Here's how the part is built. I have some questions about the finished solid (model axes, mm). Face numbers are marked on the shaded views. A direction names the side the tool comes from. Coordinates: 2 decimals unless noted, no trailing zeros. Loops run counter-clockwise (first coordinate to the right, second up) from the corner with the lowest first, then second, coordinate; pieces in that order, holes last. Notation, with made-up numbers: (69, 17.25) -> (114, 17.25) arc R23 ccw to (114, 48.25) -> close; hole circle Ø10 at (64, 33). An arc over 180 degrees is marked (long way). Use CSV: the item, a comma, the result in double quotes. Start each with the question number.
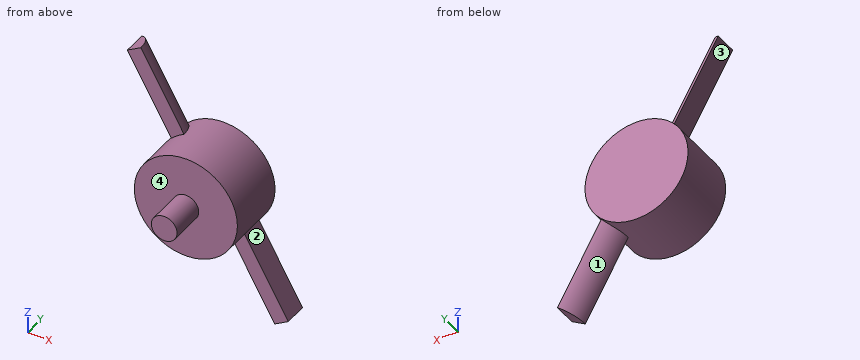
from build123d import *

# Parameters (mm, degrees)
F0_R         = 10
F1_DEPTH     = 12
F3_DEPTH     = 5
F4_T4_DEPTH  = 41.8533803035
F4_S5_R      = 10
F4_T6_DEPTH  = 25
F4_T10_DEPTH = 41.8533803035
F4_S11_R     = 10
F4_T12_DEPTH = 25
F5_R         = 2.5
F6_DEPTH     = 6.9


# Not quite as in the source:
# - a fillet or chamfer that OpenCascade refuses, or shapes differently, is made with other operations: its cross-section is extruded or revolved along the edge and cut away or added


with BuildPart() as f1:
    # F0 (on Front) → F1 (new body)
    with BuildSketch(Plane.XZ):
        Circle(F0_R)
    extrude(amount=F1_DEPTH)

    # F2 (on face) → F3 (join)
    with BuildSketch(Plane(origin=(0, 0, 0), x_dir=(-1, 0, 0), z_dir=(0, 1, 0))):
        Polygon((2.4069448783, 5), (-2.4069448783, 5), (-3, 0), (3, 0), (15.6031129395, 22), (13, 23.4912421078), align=None)
        Polygon((3, 0), (-3, 0), (-15.6031129395, -22), (-13, -23.4912421078), (-2.4069448783, -5), (2.4069448783, -5), align=None)
    extrude(amount=-F3_DEPTH)

    # F4: fillet of radius 5 on 2 edges, made by hand


with BuildPart() as f4_tool2:
    # F4_s3 → F4_t4 (new body)
    with BuildSketch(Plane(origin=(-19.5578893967, 0, 34.1402611236), x_dir=(0, 1, 0), z_dir=(0.4970807026, 0, -0.8677043132))):
        with BuildLine():
            ThreePointArc((0, -4.6031129395), (-1.4644660941, -1.0675790336), (-5, 0.3968870605))
            Line((-5, 0.3968870605), (0, 0.3968870605))
            Line((0, 0.3968870605), (0, -4.6031129395))
        make_face()
    extrude(amount=F4_T4_DEPTH)

    # F4_s5 → F4_t6 (cut, symmetric)
    with BuildSketch(Plane.XZ.offset(2.5)):
        Circle(F4_S5_R)
    extrude(amount=F4_T6_DEPTH, both=True, mode=Mode.SUBTRACT)


with BuildPart() as f1_1:
    add(f1.part)

    # F4_t1: cut F4_tool2
    add(f4_tool2.part, mode=Mode.SUBTRACT)


with BuildPart() as f4_tool8:
    # F4_s9 → F4_t10 (new body)
    with BuildSketch(Plane(origin=(19.5578893967, 0, -34.1402611236), x_dir=(0, 1, 0), z_dir=(-0.4970807026, 0, 0.8677043132))):
        with BuildLine():
            ThreePointArc((0, -4.6031129395), (-1.4644660941, -1.0675790336), (-5, 0.3968870605))
            Line((-5, 0.3968870605), (0, 0.3968870605))
            Line((0, 0.3968870605), (0, -4.6031129395))
        make_face()
    extrude(amount=F4_T10_DEPTH)

    # F4_s11 → F4_t12 (cut, symmetric)
    with BuildSketch(Plane.XZ.offset(2.5)):
        Circle(F4_S11_R)
    extrude(amount=F4_T12_DEPTH, both=True, mode=Mode.SUBTRACT)


with BuildPart() as f1_2:
    add(f1_1.part)

    # F4_t7: cut F4_tool8
    add(f4_tool8.part, mode=Mode.SUBTRACT)

    # F5 (on face) → F6 (join)
    with BuildSketch(Plane.XZ.offset(12)):
        Circle(F5_R)
    extrude(amount=F6_DEPTH)


solid = f1_2.part
1) I want a section at C-C, the plane y = -13.25. Please give me the cut outline in (x, z), plus the area to 3 significant figures.
2) Which directions (+Z, -Z, +X, -X, +Y, -Y) give clear straight access to the entire face, cutting with the end or side of a thin tool? Please do the marked faces 1, 2, 3 and 4.
3) Please list where these lines run through material, in increasing order: L1, parallel to X at y = -2.25, z = 0; L2, parallel to X at y = -6.5, z = 1; L3, parallel to Z at x = 2, y = -6. Write a range as [from, to].
4) I want a section at D-D, the plane x = 4. Please give me the cut outline in (y, z), plus the area to 3 significant figures.
5) For P1, Ø3.5, axis at x = 10.5, z = -11.5, coming from the -Y side; P2, Ø2, axis at x = 0.5, y = -14, coming from the -Z side; P3, Ø4, axis at x = 7, y = -3, coming from the +Z side, each with a flat end and sliding along its axis, tell me the tip position at first contact or that it passes through.
6) I want a section at B-B, the plane z = 0. Please give me the cut outline in (x, y), plus the area to 4 significant figures.
7) I want a section at A-A, the plane x = 0. Please give me the cut outline in (y, z).
Return value:
1,outline,"circle Ø5 at (0, 0)"
1,area,"19.6 mm²"
2,face 1,"-Z, +Y"
2,face 2,"+X, +Y, -Y"
2,face 3,"-X, +Y, -Y"
2,face 4,"-Y"
3,L1,"x = [-10, 10]"
3,L2,"x = [-9.95, 9.95]"
3,L3,"z = [-9.8, 9.8]"
4,outline,"(-12, -9.17) -> (0, -9.17) -> (0, 9.17) -> (-12, 9.17) -> close"
4,area,"220 mm²"
5,P1,"stops at y = -5"
5,P2,"stops at z = -2.5"
5,P3,"stops at z = 8.66"
6,outline,"(-10, -12) -> (-2.5, -12) -> (-2.5, -18.9) -> (2.5, -18.9) -> (2.5, -12) -> (10, -12) -> (10, 0) -> (-10, 0) -> close"
6,area,"274.5 mm²"
7,outline,"(-18.9, -2.5) -> (-12, -2.5) -> (-12, -10) -> (0, -10) -> (0, 10) -> (-12, 10) -> (-12, 2.5) -> (-18.9, 2.5) -> close"
